Part model, mm, in its own coordinate system. Face numbers are marked on the shaded views. A direction names the side the tool comes from. Coordinates: 2 decimals unless noted, no trailing zeros. Order: outer loops, then holes, each group sorted by start corner. A loop starts at its lowest first (then second) coordinate and runs counter-clockwise, first axis right, second up.
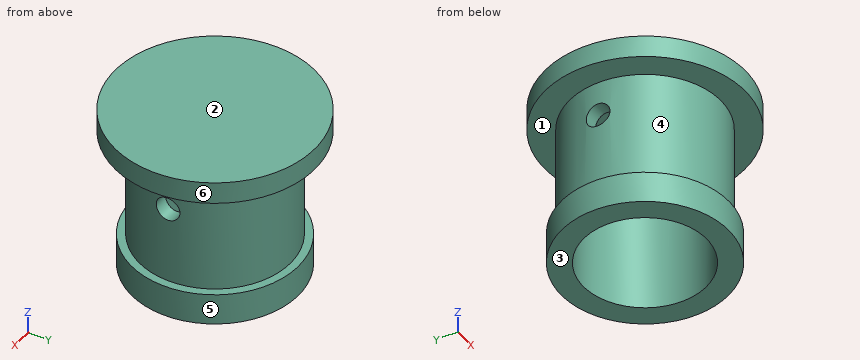
```python
from build123d import *

# Parameters (mm, degrees)
SKETCH1_R           = 5.3
SKETCH1_R_2         = 3.9
EXTRUDE1_DEPTH      = 2
SKETCH2_R           = 4.8
SKETCH2_R_2         = 3.9
EXTRUDE2_DEPTH      = 7.5
SKETCH4_R           = 0.75
EXTRUDE3_DEPTH      = 6.3
EXTRUDE3_DEPTH_BACK = 6.3
SKETCH5_R           = 6.35
EXTRUDE4_DEPTH      = 1
EXTRUDE4_DEPTH_BACK = 0.4


with BuildPart() as part:
    # Sketch1 → Extrude1 (new body)
    with BuildSketch(Plane.XY):
        Circle(SKETCH1_R)
        Circle(SKETCH1_R_2, mode=Mode.SUBTRACT)
    extrude(amount=EXTRUDE1_DEPTH)

    # Sketch2 → Extrude2 (add)
    with BuildSketch(Plane.XY.offset(2)):
        Circle(SKETCH2_R)
        Circle(SKETCH2_R_2, mode=Mode.SUBTRACT)
    extrude(amount=EXTRUDE2_DEPTH)

    # Sketch4 → Extrude3 (cut, two sides)
    with BuildSketch(Plane(origin=(0, 0, 0), x_dir=(0, 0, -1), z_dir=(1, 0, 0))) as extrude3_sk:
        with Locations((-6.9, 0)):
            Circle(SKETCH4_R)
    extrude(amount=EXTRUDE3_DEPTH, mode=Mode.SUBTRACT)
    extrude(extrude3_sk.sketch, amount=-EXTRUDE3_DEPTH_BACK, mode=Mode.SUBTRACT)

    # Sketch5 → Extrude4 (add, two sides)
    with BuildSketch(Plane.XY.offset(9.5)) as extrude4_sk:
        Circle(SKETCH5_R)
    extrude(amount=EXTRUDE4_DEPTH)
    extrude(extrude4_sk.sketch, amount=-EXTRUDE4_DEPTH_BACK)


solid = part.part
```
(1) Probe line 1 (X direction, y = 0, z = 5); line 2 (Z direction, x = 4.45, y = 0). List the from-to ranges inside material, lowest first.
(2) Slice it at A-A, the plane y = 0. Give the cut face in (x, z).
(3) Slice it at D-D, the plane z = 3.25. Give the cut face in (x, y).
(4) Slice it at B-B, the plane x = 0. Give the cut face in (y, z).
(5) Slice it at C-C, the plane z = 6.9. Give the cut face in (x, y).
(6) Pull direction Z, two halves, no side cores. Call the marked faces 1, 2, 3 and 4: +Z half, -Z half, draft (parallel to the pull), parting line (faces both ways), or undercut.
(7) Tool access for the marked faces 5 and 6: list every direction of +Z, -Z, +X, -X, +Y, -Y with a clear straight run to the whole face (end or side of a thin tool).
(8) Drop flat-ended pins along their axis: pin 1 (2.5 mm diameter, centred on x = -1, y = -0.5, fed in from -Z); pin 2 (3 mm diameter, centred on y = -2, z = 2, fed in from +X); pin 3 (1 mm diameter, centred on y = -5, z = 2, fed in from +X). Give the stop position or say it passes through.
Here are the results:
1. line 1: x = -4.8 to -3.9, 3.9 to 4.8
1. line 2: z = 0 to 6.15, 7.65 to 10.5
2. outline: (-6.35, 9.1) - (-4.8, 9.1) - (-4.8, 7.65) - (-3.9, 7.65) - (-3.9, 9.1) - (3.9, 9.1) - (3.9, 7.65) - (4.8, 7.65) - (4.8, 9.1) - (6.35, 9.1) - (6.35, 10.5) - (-6.35, 10.5) - close; (-5.3, 0) - (-3.9, 0) - (-3.9, 6.15) - (-4.8, 6.15) - (-4.8, 2) - (-5.3, 2) - close; (3.9, 0) - (5.3, 0) - (5.3, 2) - (4.8, 2) - (4.8, 6.15) - (3.9, 6.15) - close
3. outline: circle Ø9.6 at (0, 0); hole circle Ø7.8 at (0, 0)
4. outline: (-6.35, 9.1) - (-4.8, 9.1) - (-4.8, 2) - (-5.3, 2) - (-5.3, 0) - (-3.9, 0) - (-3.9, 9.1) - (3.9, 9.1) - (3.9, 0) - (5.3, 0) - (5.3, 2) - (4.8, 2) - (4.8, 9.1) - (6.35, 9.1) - (6.35, 10.5) - (-6.35, 10.5) - close
5. outline: (-4.74, -0.75) arc R4.8 ccw to (4.74, -0.75) - (3.83, -0.75) arc R3.9 cw to (-3.83, -0.75) - close; (-4.74, 0.75) - (-3.83, 0.75) arc R3.9 cw to (3.83, 0.75) - (4.74, 0.75) arc R4.8 ccw to start
6. face 1: undercut
6. face 2: +Z half
6. face 3: -Z half
6. face 4: undercut
7. face 5: -Z
7. face 6: +Z, -Z
8. pin 1: stops at z = 9.1
8. pin 2: stops at x = 5.28
8. pin 3: stops at x = 2.8
